Verification items for the finished model (mm, model axes). A direction names the side the tool comes from. Coordinates: 2 decimals unless noted, no trailing zeros. Order: outer loops, then holes, each group sorted by start corner. A loop starts at its lowest first (then second) coordinate and runs counter-clockwise, first axis right, second up. Notation, with made-up numbers: M -3.75,80 L 4.25,80 A18 ccw 4.25,89 Z; hole C 31.25,-3 d5. An arc over 180 degrees is marked long. Answer as a JSON object with one key per item and string values. Group by question number.
(1) Cross-section at A-A (x = 0). Enter the section's corners in (y, z), plus the area to 3 significant figures.
(2) Cross-section at B-B (y = 36.5). Enter the section's corners in (x, z).
(3) Gauge pin test, flat ends, axial feed: pin 1 Ø1 at (x, y) = (9, 8.5) entering from -Z; pin 2 Ø1.5 at (x, y) = (3, 57) entering from -Z; pin 3 Ø24 at (x, z) = (-6.5, 8.5) entering from -Y. Record the tip position at first contact, or that the pin passes through.
(4) Access from +Z, -Z, +X, -X, +Y, -Y to the whole of each face (thin tool, end or side, straight path). Record for faces 1 (the face through (-12, 0, -35)), 2 (the face through (36.82, 38.66, 11.59)), 3 (the face through (0, 63, 0)).
(5) Material ranges on line 1 (Z direction, x = 0, y = 15.9); line 2 (X direction, y = 13.5, z = 21), recorded low to high.
(6) Mould release check, pull along Z, two halves, no side actions. Record for faces 4 (the face through (8.44, 9.06, 38.03)), 5 (the face through (-10.7, 15, -29.2)), 6 (the face through (0, 68, 0)): released by +Z, released by -Z, zero draft, split by the parting line, or undercut.
Autodesk Inventor part; units mm, degrees
ref_plane "Work Plane1" through (0, 15, 0) normal (0, 1, 0) x (-1, 0, 0)
ref_plane "Mating Plane with Cooling Shroud" through (0, 72.6, 0) normal (0, -1, 0) x (1, 0, 0)
ref_plane "YZ Plane" through (0, 0, 0) normal (1, 0, 0) x (0, 1, 0)
sketch "Sketch1" plane through (0, 0, 0) normal (0, 1, 0) x (-1, 0, 0)
  circle A0 centre (0, 0) radius 35.1 construction
  circle A1 centre (0, 0) radius 31.4 construction
  circle A2 centre (0, 0) radius 36 construction
  circle A3 centre (0, 0) radius 27.65 construction
  circle A4 centre (0, 0) radius 32.3 construction
  circle A5 centre (0, 0) radius 31.8
  circle A6 centre (0, 0) radius 36.5
  circle A7 centre (0, 0) radius 29.8
  circle A8 centre (0, 0) radius 39.5
  dimension "d0" = 70.2
  dimension "d1" = 62.8
  dimension "d2" = 72
  dimension "d3" = 55.3
  dimension "d4" = 0.9
  dimension "d5" = 0.9
  dimension "d6" = 0.5
  dimension "d7" = 0.5
  dimension "d11" = 2
  dimension "d12" = 3
ref_plane "Work Plane1" through (0, 15, 0) normal (0, 1, 0) x (-1, 0, 0)
sketch "Sketch2" plane through (0, 15, 0) normal (0, 1, 0) x (-1, 0, 0)
  circle A0 centre (0, 0) radius 35.1 construction
  circle A1 centre (0, 0) radius 31.4 construction
  circle A2 centre (0, 0) radius 35.6
  circle A3 centre (0, 0) radius 30.9
  circle A4 centre (0, 0) radius 38.6
  circle A5 centre (0, 0) radius 28.9
  dimension "d9" = 0.5
  dimension "d10" = 0.5
  dimension "d13" = 3
  dimension "d14" = 2
loft "Loft1" add profiles "Sketch2", "Sketch1" contours A2 | A3 | A4 | A5 / A5 | A6 | A7 | A8
loft "Loft2" cut profiles "Sketch1", "Sketch2" contours A5 | A6 | A7 / A2 | A3 | A5
extrude "Extrusion1" add sketch "Sketch2" against normal up to surface (15 mm away) contours A3
sketch "Sketch3" plane through (0, 15, 0) normal (0, 1, 0) x (1, 0, 0)
  circle A0 centre (0, 0) radius 38.6
  circle A1 centre (0, 0) radius 28.9
  circle A2 centre (0, 0) radius 60.865
  dimension "d27" = 121.73
extrude "Extrusion2" add sketch "Sketch3" along normal blind 3 contours A0
ref_plane "Mating Plane with Cooling Shroud" through (0, 72.6, 0) normal (0, -1, 0) x (1, 0, 0)
ref_plane "Plane of the K flange face" through (0, 39, 0) normal (0, -1, 0) x (1, 0, 0)
sketch "Sketch4" plane through (0, 0, 0) normal (0, 1, 0) x (1, 0, 0)
  circle A0 centre (0, 0) radius 55 construction
  circle A1 centre (0, 55) radius 2.9
  circle A2 centre (0, 0) radius 39.5 construction
  circle A3 centre (0, 0) radius 60.865
  circle A4 centre (0, 0) radius 39.5
  circle A5 centre (0, 0) radius 36.5
  dimension "d30" = 110
  dimension "d31" = 5.8
  dimension "d32" = 121.73
extrude "Extrusion3" [suppressed]
extrude "Extrusion4" [suppressed]
pattern_circular "Circular Pattern1" [suppressed]
sketch "Sketch5" plane through (0, 18, 0) normal (0, 1, 0) x (1, 0, 0)
  circle A0 centre (0, 0) radius 28.9
  circle A1 centre (0, 0) radius 31.9
  dimension "d40" = 3
extrude "Extrusion5" [suppressed]
sketch "Sketch7" plane through (0, 0, 0) normal (1, 0, 0) x (0, 1, 0)
  line L0 (0, -60.865) -> (3, -60.865)
  line L1 (3, -60.865) -> (3, 60.865)
  line L2 (0, -39.5) -> (15, -38.6)
  line L3 (15, -38.6) -> (18, -38.6)
  line L4 (18, -38.6) -> (18, 38.6)
  line L5 (18, -31.9) -> (72.6, -31.9)
  line L6 (3, -60.865) -> (72.6, -60.865)
  line L7 (72.6, -60.865) -> (72.6, -31.9)
  line L8 (-14.1, 0) -> (84.6, 0)
  point P0 (0, 0)
revolve "Revolution1" [suppressed]
pattern_circular "Circular Pattern2" [suppressed]
extrude "Extrusion6" [suppressed]
pattern_circular "Circular Pattern3" [suppressed]
sketch "Sketch8" plane through (0, 72.6, 0) normal (0, 1, 0) x (-1, 0, 0)
  circle A0 centre (0, 0) radius 39.85
  point P0 (0, 0)
  dimension "d52" = 79.7
extrude "Extrusion7" [suppressed]
sketch "Sketch9" plane through (0, 55.6, 0) normal (0, 1, 0) x (1, 0, 0)
  circle A0 centre (0, 0) radius 19.55
  arc A1 (-24.4368, -20.5049) -> (24.4368, -20.5049) centre (0, 0) ccw
  circle A2 centre (0, 0) radius 31.9
  point P0 (-24.4368, -20.5049)
  dimension "d57" = 39.1
extrude "Extrusion8" [suppressed]
sketch "Sketch10" plane through (0, 57.6, 0) normal (0, 1, 0) x (1, 0, 0)
  arc A0 (6, -25.55) -> (-6, -25.55) centre (0, -25.55) ccw
  line L0 (-6, -31.9) -> (6, -31.9) construction
  circle A1 centre (0, 0) radius 31.9
  line L1 (-6, -31.9) -> (-6, -25.55)
  line L2 (6, -31.9) -> (6, -25.55)
  circle A2 centre (0, 0) radius 19.55
  point P0 (0, -31.9)
  point P1 (-6, -31.3307)
  point P2 (6, -31.3307)
  dimension "d58" = 12
  dimension "d60" = 12
extrude "Extrusion9" [suppressed]
ref_plane "Work Plane4" through (0, 67.6, 31.9) normal (0, 0, 1) x (1, 0, 0)
sketch "Sketch11" plane through (0, 67.6, 31.9) normal (0, 0, 1) x (1, 0, 0)
  circle A0 centre (0, -5) radius 3.85
  line L0 (6, 0) -> (-6, 0)
  line L1 (-6, -10) -> (-6, 0)
  point P0 (0, -67.6)
  point P1 (0, 0)
  point P2 (-6, -5)
  dimension "d63" = 7.7
extrude "Extrusion10" [suppressed]
sketch "Sketch12" plane through (0, 67.6, 0) normal (0, 1, 0) x (1, 0, 0)
  point P0 (0, 0)
sketch "Sketch13" plane through (0, 62.6, 22.9) normal (0, 0, 1) x (1, 0, 0)
  circle A0 centre (0, 0) radius 0.75
  point P0 (0, -62.6)
  dimension "d66" = 1.5
extrude "Extrusion11" [suppressed]
sketch "Sketch15" plane through (0, 55.6, 0) normal (0, -1, 0) x (1, 0, 0)
  line L0 (-3.85, 22.9) -> (3.85, 22.9)
  circle A0 centre (0, 22.9) radius 1.5
  point P0 (0, 0)
  point P1 (-0.75, 22.9)
  point P2 (0.75, 22.9)
  dimension "d71" = 3
ref_plane "Work Plane5" through (0, 66.45, 31.9) normal (0, 1, 0) x (-1, 0, 0)
extrude "Extrusion12" [suppressed]
sketch "Sketch16" plane through (0, 57.6, 0) normal (0, 1, 0) x (1, 0, 0)
  line L0 (-19.55, 0) -> (-19.55, -35)
  line L1 (-19.55, -35) -> (19.55, -35)
  line L2 (19.55, -35) -> (19.55, 0)
  circle A0 centre (0, 0) radius 19.55
  line L3 (-19.05, 0) -> (-19.05, -35)
  line L4 (19.05, 0) -> (19.05, -35)
  line L5 (-19.55, 0) -> (19.55, 0)
  point P0 (19.55, 0)
  point P1 (-19.05, -4.3932)
  point P2 (19.05, -4.3932)
  dimension "d74" = 0.5
  dimension "d75" = 0.5
  dimension "d76" = 35
extrude "Extrusion13" [suppressed]
ref_plane "Inside Plane of Lid Top" through (0, 63, 0) normal (0, -1, 0) x (1, 0, 0)
ref_plane "Top of the Dewar Neck" through (0, 38, 0) normal (0, -1, 0) x (1, 0, 0)
sketch "Sketch18" plane through (0, 18, 0) normal (0, 1, 0) x (1, 0, 0)
  circle A0 centre (0, 0) radius 38.6
  circle A1 centre (0, 0) radius 28.9
extrude "Extrusion14" add sketch "Sketch18" along normal up to surface (45 mm away)
sketch "Sketch19" plane through (0, 63, 0) normal (0, 1, 0) x (1, 0, 0)
  circle A0 centre (0, 0) radius 38.6
extrude "Extrusion15" add sketch "Sketch19" along normal blind 5
fillet "Fillet1" radius 5 1 edges at (-38.6, 68, 0)
fillet "Fillet2" radius 5 1 edges at (-28.9, 63, 0)
properties part number "Pope8697-Adapter_3DPrint"
Taken from the geometry:
{
 "1": {"outline": "M 0,-39.5 L 15,-38.6 L 63,-38.6 A5 ccw 68,-33.6 L 68,33.6 A5 ccw 63,38.6 L 15,38.6 L 0,39.5 L 0,36.5 L 15,35.6 L 15,30.9 L 0,30.9 L 0,28.9 L 58,28.9 A5 cw 63,23.9 L 63,-23.9 A5 cw 58,-28.9 L 0,-28.9 L 0,-30.9 L 15,-30.9 L 15,-35.6 L 0,-36.5 Z", "area": "1,470 mm²"},
 "2": {"outline": "C 0,0 d77.2; hole C 0,0 d57.8"},
 "3": {"pin 1": "stops at z = -38.06", "pin 2": "stops at z = -38.53", "pin 3": "stops at y = 63"},
 "4": {"face 1": "+Z, -Z, +X, -X, -Y", "face 2": "+Y", "face 3": "-Y"},
 "5": {"line 1": "z = -38.6 to -28.9, 28.9 to 38.6", "line 2": "x = -32.49 to -28.86, -22.67 to -19.85, 19.85 to 22.67, 28.86 to 32.49"},
 "6": {"face 4": "split by the parting line", "face 5": "undercut", "face 6": "zero draft"}
}
